Solid Edge part; units mm, degrees
sketch "Sketch1" plane through (0, 0, 0) normal (0, -1, 0) x (1, 0, 0)
  line L0 (-500, -15) -> (500, -15)
  line L1 (500, -15) -> (500, 15)
  line L2 (500, 15) -> (-500, 15)
  line L3 (-500, 15) -> (-500, -15)
extrude "Protrusion1" add sketch "Sketch1" along normal mid plane 20
fillet "Round_1" radius 15 2 edges at (-500, 0, 15) (-500, 0, -15)
sketch "Sketch2" plane through (0, -10, 0) normal (0, -1, 0) x (1, 0, 0)
  circle A0 centre (-485, 0) radius 10
extrude "ExtrudedCutout_1" cut sketch "Sketch2" against normal blind 60
sketch "Sketch3" plane through (0, -10, 0) normal (0, -1, 0) x (1, 0, 0)
  line L0 (-395, 7) -> (-384, 7)
  line L1 (-384, -7) -> (-395, -7)
  arc A0 (-384, 7) -> (-384, -7) centre (-384, 0) cw
  arc A1 (-395, -7) -> (-395, 7) centre (-395, 0) cw
extrude "ExtrudedCutout_2" cut sketch "Sketch3" against normal blind 20
sketch "Sketch4" plane through (0, -10, 0) normal (0, -1, 0) x (1, 0, 0)
  line L0 (-395, 7.71) -> (-384, 7.71)
  line L1 (-384, 7.71) -> (-384, -7.71)
  line L2 (-395, -7.71) -> (-384, -7.71)
  line L3 (-395, 7.71) -> (-395, -7.71)
extrude "ExtrudedCutout_3" cut sketch "Sketch4" against normal blind 20
sketch "Sketch5" plane through (0, 10, 0) normal (0, 1, 0) x (1, 0, 0)
  circle A0 centre (-470.3635, 6.2542) radius 2.5
extrude "ExtrudedCutout_6" cut sketch "Sketch5" against normal blind 20
sketch "Sketch6" plane through (-0.5, -10, 0) normal (0, -1, 0) x (-1, 0, 0)
  line L0 (-499.5, 15) -> (-500.5, 15)
  line L1 (-500.5, 15) -> (-500.5, 14)
  line L2 (-500.5, 14) -> (-499.5, 15)
  line L3 (-500.5, -14) -> (-500.5, -15)
  line L4 (-500.5, -15) -> (-499.5, -15)
  line L5 (-499.5, -15) -> (-500.5, -14)
extrude "ExtrudedCutout_8" cut sketch "Sketch6" along normal mid plane 240
sketch "Sketch7" plane through (500, 0, 0) normal (1, 0, 0) x (0, 0, -1)
  line L0 (-15, -10) -> (15, -10)
  line L1 (15, -10) -> (15, 10)
  line L2 (15, 10) -> (-15, 10)
  line L3 (-15, 10) -> (-15, -10)
extrude "ExtrudedProtrusion_2" add sketch "Sketch7" along normal mid plane 15
sketch "Sketch8" plane through (11.25, 0, -15) normal (0, 0, -1) x (-1, 0, 0)
  line L0 (-495.25, 10) -> (-496.25, 10)
  line L1 (-496.25, 10) -> (-496.25, 9)
  line L2 (-496.25, 9) -> (-495.25, 10)
  line L3 (-495.25, -10) -> (-496.25, -10)
  line L4 (-496.25, -10) -> (-496.25, -9)
  line L5 (-496.25, -9) -> (-495.25, -10)
extrude "ExtrudedCutout_9" cut sketch "Sketch8" along normal mid plane 80
sketch "Sketch9" plane through (3.25, -10, 0) normal (0, -1, 0) x (-1, 0, 0)
  line L0 (-504.25, 15) -> (-504.25, 14)
  line L1 (-504.25, 14) -> (-503.25, 15)
  line L2 (-503.25, 15) -> (-504.25, 15)
  line L3 (-504.25, -15) -> (-504.25, -14)
  line L4 (-504.25, -14) -> (-503.25, -15)
  line L5 (-503.25, -15) -> (-504.25, -15)
extrude "ExtrudedCutout_10" cut sketch "Sketch9" along normal mid plane 40
properties material "Steel - Stainless:1.4301 , X5CrNi18-10"
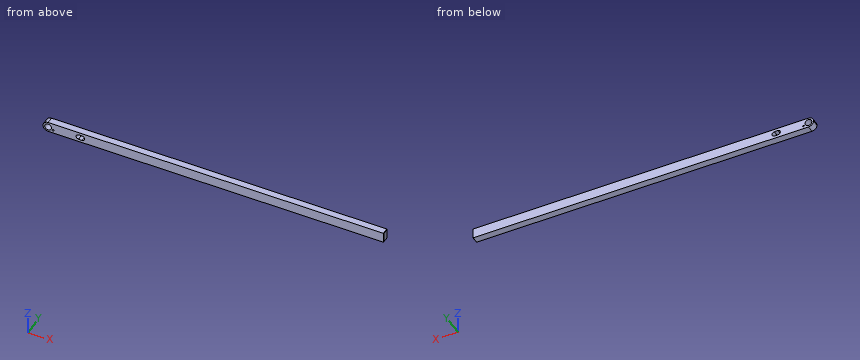
Input: part model. Units: mm. Frame: model coordinates. Give positions to 0.01 mm unless a question says otherwise; leave off trailing zeros. Answer as a JSON object with one key per item and string values. Group by question number.
Item 1: Pin query (flat end, axial travel): P1, Ø5, axis at y = 4, z = -3.5, coming from the -X side; P2, Ø0.6, axis at y = 4.5, z = 7.5, coming from the -X side. Return the tip coordinate at first contact, or that it passes through.
Item 2: Cut plane A-A, the plane y = -5.75. State how many separate pieces and enclosed holes the cut face has, and give its area (3 significant figures).
Item 3: Line query: probe 1 along X at (y, z) = (6.5, 1.5); probe 2 along X at (y, z) = (2.25, 2); probe 3 along Z at (x, y) = (-485, -3.5). Output: solid intervals per line, ascending.
Checks:
{
 "1": {"P1": "stops at x = -499.97", "P2": "stops at x = -498.16"},
 "2": {"separate pieces": "1", "enclosed holes": "3", "area": "29,500 mm²"},
 "3": {"probe 1": "x = -499.92 to -494.89, -475.11 to -401.84, -377.16 to 507.5", "probe 2": "x = -499.87 to -494.8, -475.2 to -401.71, -377.29 to 507.5", "probe 3": "z = -15 to -10, 10 to 15"}
}
